Autodesk Inventor part; units mm, degrees
ref_plane "BODY_N_XY" through (82, 0, 0) normal (0, 0, -1) x (1, 0, 0)
ref_plane "BODY_N_YZ" through (82, 0, 0) normal (1, 0, 0) x (0, -1, 0)
ref_plane "BODY_N_ZX" through (82, 0, 0) normal (0, -1, 0) x (0, 0, -1)
sketch "Sketch_8" plane through (0, 0, 0) normal (0, 0, 1) x (1, 0, 0)
  line L0 (0, 0) -> (-8, 0)
  line L1 (-8, 0) -> (-8, 4.3865)
  line L2 (-8, 4.3865) -> (-7.3865, 5)
  line L3 (-7.3865, 5) -> (0, 5)
  line L4 (0, 5) -> (0, 0)
  line L5 (0, 0) -> (-8, 0)
revolve "Revolution1" add sketch "Sketch_8" angle 360 about axis through (0, 0, 0) along (1, 0, 0)
thread "Thread1"
sketch "Sketch_9" plane through (0, 0, 0) normal (1, 0, 0) x (0, 0, -1)
  line L0 (-9.15, 4.0345) -> (-9.15, -4.0345)
  arc A0 (-9.15, -4.0345) -> (-4.0345, -9.15) centre (0, 0) ccw
  line L1 (-4.0345, -9.15) -> (4.0345, -9.15)
  arc A1 (4.0345, -9.15) -> (9.15, -4.0345) centre (0, 0) ccw
  line L2 (9.15, -4.0345) -> (9.15, 4.0345)
  arc A2 (9.15, 4.0345) -> (4.0345, 9.15) centre (0, 0) ccw
  line L3 (4.0345, 9.15) -> (-4.0345, 9.15)
  arc A3 (-4.0345, 9.15) -> (-9.15, 4.0345) centre (0, 0) ccw
extrude "Extrusion1" add sketch "Sketch_9" along normal blind 12.5
sketch "Sketch_11" plane through (12.5, 0, 0) normal (1, 0, 0) x (0, 0, -1)
  circle A0 centre (0, 0) radius 8.7
extrude "Extrusion2" add sketch "Sketch_11" along normal blind 50
sketch "Sketch_10" plane through (62.5, 0, 0) normal (1, 0, 0) x (0, 0, -1)
  line L0 (-9.15, 4.0345) -> (-9.15, -4.0345)
  arc A0 (-9.15, -4.0345) -> (-4.0345, -9.15) centre (0, 0) ccw
  line L1 (-4.0345, -9.15) -> (4.0345, -9.15)
  arc A1 (4.0345, -9.15) -> (9.15, -4.0345) centre (0, 0) ccw
  line L2 (9.15, -4.0345) -> (9.15, 4.0345)
  arc A2 (9.15, 4.0345) -> (4.0345, 9.15) centre (0, 0) ccw
  line L3 (4.0345, 9.15) -> (-4.0345, 9.15)
  arc A3 (-4.0345, 9.15) -> (-9.15, 4.0345) centre (0, 0) ccw
extrude "Extrusion3" add sketch "Sketch_10" along normal blind 27.5
sketch "Sketch5" plane through (0, 9.15, 4.0345) normal (0, 1, 0) x (1, 0, 0)
  point P0 (8, 4.0345)
hole "Hole1" at (8, 9.15, 0) direction (0, -1, 0) diameter 5 depth 5 tip angle 120
sketch "Sketch6" plane through (62.5, 9.15, 4.0345) normal (0, 1, 0) x (1, 0, 0)
  point P0 (4.5, 4.0345)
hole "Hole2" at (67, 9.15, 0) direction (0, -1, 0) diameter 5 depth 5 tip angle 120
sketch "Sketch_16" plane through (0, 0, 0) normal (0, 0, 1) x (1, 0, 0)
  line L0 (42.5, 0) -> (-8, 0)
  line L1 (-8, 0) -> (-8, 2.5)
  line L2 (-8, 2.5) -> (12.5, 2.5)
  line L3 (12.5, 2.5) -> (12.5, 8)
  line L4 (12.5, 8) -> (42.5, 8)
  line L5 (42.5, 8) -> (42.5, 0)
  line L6 (42.5, 0) -> (-8, 0)
revolve "Revolution2" cut sketch "Sketch_16" angle 360 about axis through (42.5, 0, 0) along (1, 0, 0)
sketch "Sketch_3" plane through (0, 0, 0) normal (0, 1, 0) x (-1, 0, 0)
  line L0 (-72, 3.25) -> (-90, 3.25)
  line L1 (-90, 3.25) -> (-90, -3.25)
  line L2 (-90, -3.25) -> (-72, -3.25)
  line L3 (-72, -3.25) -> (-72, 3.25)
extrude "Extrusion4" cut sketch "Sketch_3" along normal mid plane 18.3
sketch "Sketch_13" plane through (0, 0, 0) normal (0, 0, 1) x (1, 0, 0)
  circle A0 centre (82, 0) radius 2.5
extrude "Extrusion5" cut sketch "Sketch_13" along normal mid plane 18.3
ref_plane "BODY_N_XY" through (82, 0, 0) normal (0, 0, -1) x (1, 0, 0)
ref_plane "BODY_N_YZ" through (82, 0, 0) normal (1, 0, 0) x (0, -1, 0)
ref_plane "BODY_N_ZX" through (82, 0, 0) normal (0, -1, 0) x (0, 0, -1)
ref_plane "BODY_PIN_XY" through (82, 0, 0) normal (-1, 0, 0) x (0, 0, -1)
ref_plane "BODY_PIN_YZ" through (82, 0, 0) normal (0, 0, -1) x (0, -1, 0)
ref_plane "BODY_PIN_ZX" through (82, 0, 0) normal (0, -1, 0) x (-1, 0, 0)
ref_plane "NUT2_XY" through (72, 0, 0) normal (1, 0, 0) x (0, 0, -1)
ref_plane "NUT2_YZ" through (72, 0, 0) normal (0, 0, -1) x (0, 1, 0)
ref_plane "NUT2_ZX" through (72, 0, 0) normal (0, 1, 0) x (1, 0, 0)
ref_plane "SW1_XY" through (17.5, 0, 0) normal (1, 0, 0) x (0, 0, -1)
ref_plane "SW1_YZ" through (17.5, 0, 0) normal (0, 0, -1) x (0, 1, 0)
ref_plane "SW1_ZX" through (17.5, 0, 0) normal (0, 1, 0) x (1, 0, 0)
ref_plane "SW2_XY" through (57.5, 0, 0) normal (-1, 0, 0) x (0, 0, -1)
ref_plane "SW2_YZ" through (57.5, 0, 0) normal (0, 0, -1) x (0, -1, 0)
ref_plane "SW2_ZX" through (57.5, 0, 0) normal (0, -1, 0) x (-1, 0, 0)
ref_plane "SW_R1_XY" through (17.5, -14.15, 0) normal (1, 0, 0) x (0, 0, -1)
ref_plane "SW_R1_YZ" through (17.5, -14.15, 0) normal (0, 0, -1) x (0, 1, 0)
ref_plane "SW_R1_ZX" through (17.5, -14.15, 0) normal (0, 1, 0) x (1, 0, 0)
ref_plane "SW_R2_XY" through (57.5, -14.15, 0) normal (-1, 0, 0) x (0, 0, -1)
ref_plane "SW_R2_YZ" through (57.5, -14.15, 0) normal (0, 0, -1) x (0, -1, 0)
ref_plane "SW_R2_ZX" through (57.5, -14.15, 0) normal (0, -1, 0) x (-1, 0, 0)
ref_plane "body_XY" through (0, 0, 0) normal (-1, 0, 0) x (0, 0, -1)
ref_plane "body_YZ" through (0, 0, 0) normal (0, 0, -1) x (0, -1, 0)
ref_plane "body_ZX" through (0, 0, 0) normal (0, -1, 0) x (-1, 0, 0)
properties part number "CJ2D16-25Z(1_1)_BODY"
Source: CAD feature listing. Evaluate the final solid. Frame: model axes, mm. A direction names the side the tool comes from. Round coordinates to 2 decimals unless told otherwise and drop trailing zeros. Write each loop counter-clockwise with the first axis right and the second up, starting at its lowest first coordinate (ties: lowest second). Pieces come first, ordered by that corner, then holes. Notation, with made-up numbers: M 75.25,48.5 L 102.25,48.5 A29 cw 102.25,77.5 Z; hole C 47.25,-26.5 d5. An arc over 180 degrees is marked long. Use CSV: the item, a comma, the result in double quotes. Start each with the question number.
Q1. Cut plane B-B on y = -6.75. Output: boundary loops of the cut face in (x, z).
Q2. Pull-direction query (Y, two-part tool) for faces 1 (the face through (62.5, -9, 1)), 2 (the face through (6.16, -7.03, -7.11)), 3 (the face through (2.39, -0.54, -2.44)); classes: +Y half, -Y half, draft (parallel to the pull), parting line (faces both ways), or undercut.
Q3. Access query for faces 4 (the face through (6.16, -7.11, 7.03)), 5 (the face through (27.71, -1.73, -7.81)), 6 (the face through (79, 0, 3.25)). Directions: +Z, -Z, +X, -X, +Y, -Y. A direction counts if a zero-diameter tool reaches every point of the face in a straight line with its end or side. Return the directions, or none.
Q4. First-contact query: P1, Ø10, axis at x = 76.5, z = 6, coming from the +Y side; P2, Ø6, axis at x = 50, y = 0.5, coming from the -Z side; P3, Ø1, axis at y = 7, z = 3, coming from the -X side; P4, Ø4, axis at x = 61, z = 5.5, coming from the +Y side. Flat tips, straight axial feed; report the tip coordinate or a pass-through.
Q5. Cut plane A-A on x = 82. Output: boundary loops of the cut face in (y, z), plus the area to 3 significant figures.
Q6. Line query: line 1 (X direction, y = 7.15, z = 0); line 2 (X direction, y = -3, z = -6.25); line 3 (X direction, y = -5, z = 8.25). Output: solid intervals per line, ascending. Write a range as from..to.
Q7. Cut plane D-D on x = 14.5. Output: boundary loops of the cut face in (y, z), plus the area to 3 significant figures.
Q8. Cut plane C-C on y = 0. Count the separate pieces of the cut face and the enclosed holes in it, plus the area to 3 significant figures.
Results found:
1,outline,"M 0,-7.38 L 12.5,-7.38 L 12.5,-5.49 L 62.5,-5.49 L 62.5,-7.38 L 90,-7.38 L 90,-3.25 L 72,-3.25 L 72,3.25 L 90,3.25 L 90,7.38 L 62.5,7.38 L 62.5,5.49 L 12.5,5.49 L 12.5,7.38 L 0,7.38 Z; hole M 12.5,-4.29 L 42.5,-4.29 L 42.5,4.29 L 12.5,4.29 Z"
2,face 1,"draft"
2,face 2,"-Y half"
2,face 3,"undercut"
3,face 4,"+Z, +X, -X, -Y"
3,face 5,"none"
3,face 6,"+X, +Y, -Y"
4,P1,"y = 9.15"
4,P2,"z = -8.7"
4,P3,"x = 0"
4,P4,"y = 9.09"
5,outline,"M -9.15,-4.03 A10 ccw -4.03,-9.15 L -2.5,-9.15 L -2.5,-3.25 L -9.15,-3.25 Z; M -9.15,3.25 L -2.5,3.25 L -2.5,9.15 L -4.03,9.15 A10 ccw -9.15,4.03 Z; M 2.5,-9.15 L 4.03,-9.15 A10 ccw 9.15,-4.03 L 9.15,-3.25 L 2.5,-3.25 Z; M 2.5,3.25 L 9.15,3.25 L 9.15,4.03 A10 ccw 4.03,9.15 L 2.5,9.15 Z"
5,area,"118 mm^2"
6,line 1,"0..5.5, 10.5..12.5, 42.5..64.5, 69.5..72"
6,line 2,"0..12.5, 42.5..90"
6,line 3,"0..12.5, 62.5..90"
7,outline,"C 0,0 d17.4; hole C 0,0 d16"
7,area,"36.7 mm^2"
8,separate pieces,"3"
8,enclosed holes,"0"
8,area,"923 mm^2"
